Part model, mm, in its own coordinate system. A direction names the side the tool comes from. Give positions to 0.01 mm unless a question says otherwise; leave off trailing zeros. Write each loop counter-clockwise with the first axis right and the second up, starting at its lowest first coordinate (ties: lowest second). Pieces come first, ordered by that corner, then holes. Notation, with made-up numbers: M -17.75,60 L 21.25,60 A18 cw 21.25,95 Z; hole C 45,17.5 d10. An arc over 180 degrees is marked long. Use a Markdown table: item, result.
```python
from build123d import *

# Parameters (mm, degrees)
F0_W     = 26
F0_H     = 26
F0_W_2   = 18
F0_H_2   = 18
F0_W_3   = 16
F0_H_3   = 16
F1_DEPTH = 2
F2_DEPTH = 0.5
F4_D     = 2.7
F4_DEPTH = 3.5
F4_TIP   = 0.8111618357


with BuildPart() as f1:
    # F0 (on Top) → F1 (new body)
    with BuildSketch(Plane.XY):
        Rectangle(F0_W, F0_H)
        Rectangle(F0_W_2, F0_H_2, mode=Mode.SUBTRACT)
        Rectangle(F0_W_2, F0_H_2)
        Rectangle(F0_W_3, F0_H_3, mode=Mode.SUBTRACT)
    extrude(amount=F1_DEPTH)

    # F0 (on Top) → F2 (cut)
    with BuildSketch(Plane.XY):
        Rectangle(F0_W_2, F0_H_2)
        Rectangle(F0_W_3, F0_H_3, mode=Mode.SUBTRACT)
    extrude(amount=F2_DEPTH, mode=Mode.SUBTRACT)

    # F4
    with Locations(Plane(origin=(0, 0, 0), x_dir=(1, 0, 0), z_dir=(0, 0, -1))):
        with Locations((-10.5, 10.5), (10.5, 10.5), (10.5, -10.5), (-10.5, -10.5)):
            Hole(F4_D / 2, depth=F4_DEPTH)
            with Locations((0, 0, -(F4_DEPTH + F4_TIP / 2))):  # 118° drill point
                Cone(0, F4_D / 2, F4_TIP, mode=Mode.SUBTRACT)


solid = f1.part
```
1. Drop a flat-ended pin along its axis: P1, Ø5, axis at x = -2.5, y = -7, coming from the -Z side. Give the stop position or say it passes through.
Findings below:
| item | result |
|---|---|
| P1 | z = 0 |
2. Two-plate mould, pull along Y, no slides. Class faces 1 (the flat face through (0, 13, 1)), 2 (the flat face through (-13, 0, 1)), 3 (the flat face through (8, 0, 1)), 4 (the flat face through (-8, 0, 1)): released by +Y, released by -Y, zero draft, split by the parting line, or undercut.
Findings below:
| item | result |
|---|---|
| face 1 | released by +Y |
| face 2 | zero draft |
| face 3 | undercut |
| face 4 | undercut |
3. Tool access for faces 5 (the flat face through (-12, 0, 0)), 6 (the flat face through (0, -8, 1)): list every direction of +Z, -Z, +X, -X, +Y, -Y with a clear straight run to the whole face (end or side of a thin tool).
Findings below:
| item | result |
|---|---|
| face 5 | -Z, +X, -X, +Y, -Y |
| face 6 | +Z, -Z |
4. Drill centre lines: L1, parallel to Y at x = 10.5, z = 1.1; L2, parallel to X at y = 3, z = 0.1. Where is each one in solid material? Low to high.
Findings below:
| item | result |
|---|---|
| L1 | -13 to -11.85, -9.15 to 9.15, 11.85 to 13 |
| L2 | -13 to -9, 9 to 13 |
5. Cut at A-A, the plane y = 10.5. Give the cut face in (x, z).
Findings below:
| item | result |
|---|---|
| outline | M -13,0 L -11.85,0 L -11.85,2 L -13,2 Z; M -9.15,0 L 9.15,0 L 9.15,2 L -9.15,2 Z; M 11.85,0 L 13,0 L 13,2 L 11.85,2 Z |
6. Cut at B-B, the plane x = 2.5. Give the cut face in (y, z).
Findings below:
| item | result |
|---|---|
| outline | M -13,0 L -9,0 L -9,0.5 L -8,0.5 L -8,2 L -13,2 Z; M 8,0.5 L 9,0.5 L 9,0 L 13,0 L 13,2 L 8,2 Z |
7. Cut at C-C, the plane z = 0.8. Give the cut face in (x, y), then the cut area to 3 significant figures.
Findings below:
| item | result |
|---|---|
| outline | M -13,-13 L 13,-13 L 13,13 L -13,13 Z; hole C -10.5,-10.5 d2.7; hole C -10.5,10.5 d2.7; hole M -8,-8 L 8,-8 L 8,8 L -8,8 Z; hole C 10.5,-10.5 d2.7; hole C 10.5,10.5 d2.7 |
| area | 397 mm2 |
